Could you check a few things on this model? Use its own coordinates, in mm. Face numbers are marked on the shaded views. A direction names the side the tool comes from. Give positions to 0.01 mm unless a question says otherwise; leave off trailing zeros. Write each loop counter-clockwise with the first axis right and the second up, starting at its lowest first coordinate (ties: lowest second). Pieces come first, ordered by that corner, then holes. Notation, with made-up numbers: (-7, 57.25) - (14, 57.25) arc R20 ccw to (14, 94.25) - close; hole circle Ø9 at (-29.75, 59.25). An arc over 180 degrees is marked (long way). Use one line per item in the form item = value.
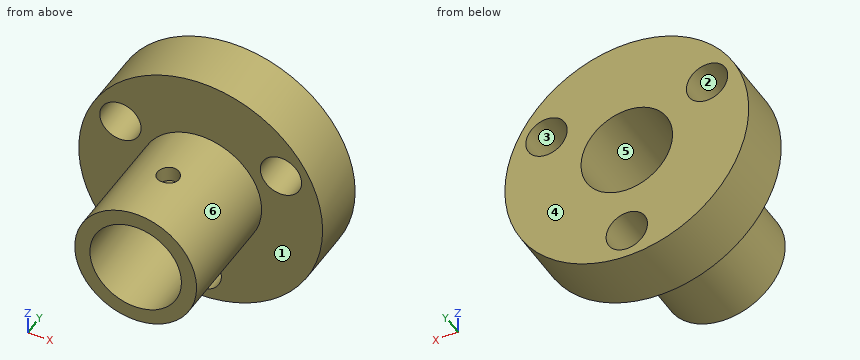
```python
from build123d import *

# Parameters (mm, degrees)
SKETCH1_R                        = 6.35
BOSS_EXTRUDE1_DEPTH              = 12.7
SKETCH2_R                        = 12.7
BOSS_EXTRUDE2_DEPTH              = 6.35
SKETCH3_R                        = 4.76758
CUT_EXTRUDE1_DEPTH               = 20.05
F_18_0_1695_DIAMETER_HOLE1_D     = 4.3053
F_18_0_1695_DIAMETER_HOLE1_DEPTH = 25.4
F_18_0_1695_DIAMETER_HOLE1_TIP   = 1.293442612


with BuildPart() as part:
    # Sketch1 → Boss-Extrude1 (new body)
    with BuildSketch(Plane(origin=(0, 0, 0), x_dir=(1, 0, 0), z_dir=(0, 1, 0))):
        Circle(SKETCH1_R)
    extrude(amount=BOSS_EXTRUDE1_DEPTH)

    # Sketch2 → Boss-Extrude2 (add)
    with BuildSketch(Plane(origin=(0, 12.7, 0), x_dir=(1, 0, 0), z_dir=(0, 1, 0))):
        Circle(SKETCH2_R)
    extrude(amount=BOSS_EXTRUDE2_DEPTH)

    # Sketch3 → Cut-Extrude1 (cut, through all)
    with BuildSketch(Plane(origin=(0, 19.05, 0), x_dir=(1, 0, 0), z_dir=(0, 1, 0))):
        Circle(SKETCH3_R)
    extrude(amount=-CUT_EXTRUDE1_DEPTH, mode=Mode.SUBTRACT)

    # #18 (0.1695) Diameter Hole1
    with Locations(Plane(origin=(0, 19.05, 0), x_dir=(1, 0, 0), z_dir=(0, 1, 0))):
        with Locations((0, 9.652), (-8.358877197, -4.826), (8.358877197, -4.826)):
            Hole(F_18_0_1695_DIAMETER_HOLE1_D / 2, depth=F_18_0_1695_DIAMETER_HOLE1_DEPTH)
            with Locations((0, 0, -(F_18_0_1695_DIAMETER_HOLE1_DEPTH + F_18_0_1695_DIAMETER_HOLE1_TIP / 2))):  # 118° drill point
                Cone(0, F_18_0_1695_DIAMETER_HOLE1_D / 2, F_18_0_1695_DIAMETER_HOLE1_TIP, mode=Mode.SUBTRACT)

    # Sketch8 → #43 (0.089) Diameter Hole1 (revolve, cut)
    with BuildSketch(Plane(origin=(0, 6.35, 0), x_dir=(0, 1, 0), z_dir=(1, 0, 0))):
        Polygon((0, 0), (0, 26.079152758), (1.1303, 25.4), (1.1303, 0), align=None)
    revolve(axis=Axis((0, 6.35, -6.35), (0, 0, 1)), mode=Mode.SUBTRACT)


solid = part.part
```
1. Imagine slicing it at C-C, the plane x = 9.75. List the corners of the cut face in (y, z) for me, and give its area (3 significant figures).
Response values:
outline = (12.7, -8.14) - (19.05, -8.14) - (19.05, 3.18) - (12.7, 3.18) - close; (12.7, 6.47) - (19.05, 6.47) - (19.05, 8.14) - (12.7, 8.14) - close
area = 82.5 mm²
2. Imagine slicing it at D-D, the plane z = 3.25. List the corners of the cut face in (x, y) for me, and give its area (3 significant figures).
Response values:
outline = (-12.28, 12.7) - (-9.83, 12.7) - (-9.83, 19.05) - (-12.28, 19.05) - close; (-6.89, 12.7) - (-5.46, 12.7) - (-5.46, 0) - (-3.49, 0) - (-3.49, 19.05) - (-6.89, 19.05) - close; (3.49, 0) - (5.46, 0) - (5.46, 12.7) - (6.89, 12.7) - (6.89, 19.05) - (3.49, 19.05) - close; (9.83, 12.7) - (12.28, 12.7) - (12.28, 19.05) - (9.83, 19.05) - close
area = 124 mm²
3. Which directions (+Z, -Z, +X, -X, +Y, -Y) give clear straight access to the entire face, cutting with the end or side of a thin tool? Please do the marked faces 1 and 2.
Response values:
face_1 = -Y
face_2 = +Y, -Y
4. Imagine slicing it at B-B, the plane z = 0. List the corners of the cut face in (x, y) for me, and give its area (3 significant figures).
Response values:
outline = (-12.7, 12.7) - (-6.35, 12.7) - (-6.35, 0) - (-4.77, 0) - (-4.77, 19.05) - (-12.7, 19.05) - close; (4.77, 0) - (6.35, 0) - (6.35, 12.7) - (12.7, 12.7) - (12.7, 19.05) - (4.77, 19.05) - close
area = 141 mm²
5. If I drill on line 1 (Z direction, x = 0, y = 14); line 2 (X direction, y = 15.5, z = 3.25); line 3 (Y direction, x = 0, z = 5.3), over which ranges is the centre line in solid material (lowest first)? Write a range as from..to.
Response values:
line_1 = -12.7..-11.8, -7.5..-4.77, 4.77..12.7
line_2 = -12.28..-9.83, -6.89..-3.49, 3.49..6.89, 9.83..12.28
line_3 = 0..5.22, 7.48..19.05
6. Imagine slicing it at A-A, the plane x = 0. List the corners of the cut face in (y, z) for me, and give its area (3 significant figures).
Response values:
outline = (0, -6.35) - (12.7, -6.35) - (12.7, -7.5) - (19.05, -7.5) - (19.05, -4.77) - (0, -4.77) - close; (0, 4.77) - (5.22, 4.77) - (5.22, 6.35) - (0, 6.35) - close; (7.48, 4.77) - (19.05, 4.77) - (19.05, 12.7) - (12.7, 12.7) - (12.7, 6.35) - (7.48, 6.35) - close; (12.7, -12.7) - (19.05, -12.7) - (19.05, -11.8) - (12.7, -11.8) - close
area = 110 mm²
7. If we mould it in two halves opening along X, with no side actions, what happens to the marked faces 3, 4, 5 and 6? For each: pulls with the +X half, pulls with the -X half, needs draft (parallel to the pull), parting line crosses it, or undercut.
Response values:
face_3 = undercut
face_4 = needs draft
face_5 = undercut
face_6 = parting line crosses it
8. For pin 1 (3 mm diameter, centred on x = -8.5, z = -2.5, fed in from -Y); pin 2 (5 mm diameter, centred on y = 15, z = 5, fed in from +X); pin 3 (6 mm diameter, centred on y = 15.5, z = 6.5, fed in from -X); pin 4 (2.5 mm diameter, centred on x = 0, z = -9.652, fed in from -Y), each with a flat end and sliding along its axis, tell me the tip position at first contact or that it passes through.
Response values:
pin_1 = 12.7
pin_2 = 12.45
pin_3 = -12.21
pin_4 = through
